Can you work these out from the drawing? Everything is in mm from the part's minimum corner. Give positions to 0.01 mm unless a question says otherwise; leave off trailing zeros. Order: outer loops, then holes, each group sorted by start corner. A loop starts at its lowest first (then second) coordinate and runs counter-clockwise, first axis right, second up. Notation, with made-up numbers: M -29.5,54.25 L -4.5,54.25 A25 ccw -4.5,80.25 Z; hole C 16.25,73.5 d4. An arc over 180 degrees is marked long. Answer as a JSON object with one key per item and string values.
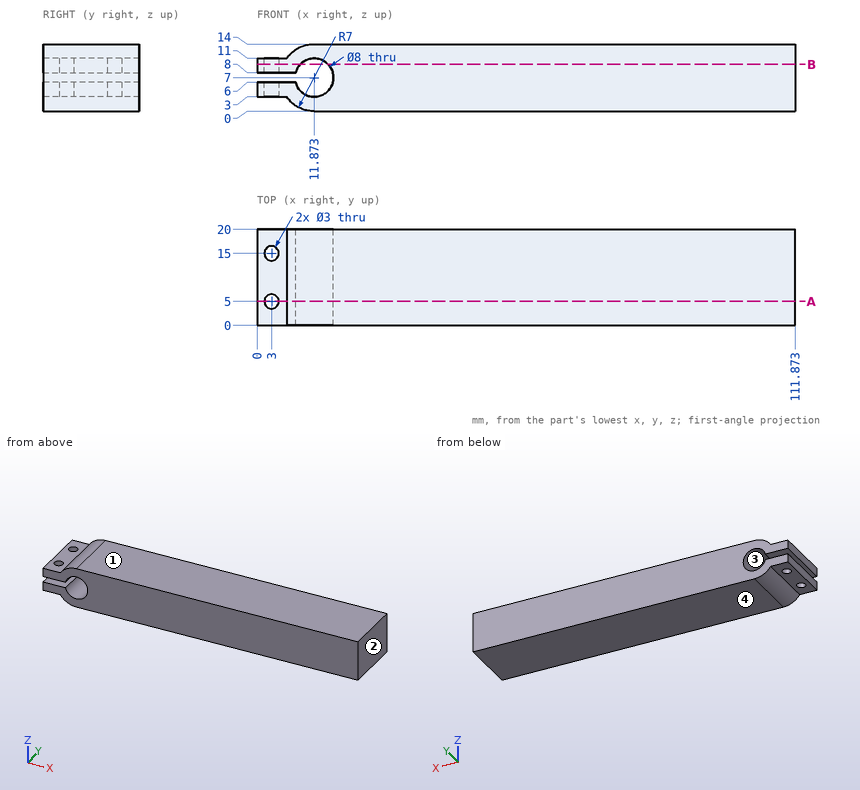
1) I need wall thicknesses on L1, parallel to Y at x = 3, z = 9.65; L2, parallel to Z at x = 14, y = 18.75; L3, parallel to X at y = 13.25, z = 7. Which ranges of each line are inside material? Lowest first, please.
Results found:
{"L1": "y = 0 to 3.5, 6.5 to 13.5, 16.5 to 20", "L2": "z = 0 to 3.61, 10.39 to 14", "L3": "x = 15.87 to 111.87"}
2) Thinking about a two-plate mould opening in Z: for the marked faces 1, 2, 3 and 4, which applies, pulls with the +Z half, pulls with the -Z half, needs draft (parallel to the pull), parting line crosses it, or undercut?
Results found:
{"face 1": "pulls with the +Z half", "face 2": "needs draft", "face 3": "undercut", "face 4": "pulls with the -Z half"}
3) I want a section at B-B on z = 9.75. Write out the boundary of the cut face in (x, y), and give its area (3 significant figures).
Results found:
{"outline": "M 0,0 L 8.97,0 L 8.97,20 L 0,20 Z; M 14.78,0 L 111.87,0 L 111.87,20 L 14.78,20 Z; hole C 3,5 d3; hole C 3,15 d3", "area": "2,110 mm²"}
4) I want a section at A-A on y = 5. Write out the boundary of the cut face in (x, z), and give its area (3 significant figures).
Results found:
{"outline": "M 0,3 L 1.5,3 L 1.5,6 L 0,6 Z; M 0,8 L 1.5,8 L 1.5,11 L 0,11 Z; M 4.5,3 L 6.13,3 A7 ccw 11.87,0 L 111.87,0 L 111.87,14 L 11.87,14 A7 ccw 6.13,11 L 4.5,11 L 4.5,8 L 8,8 A4 cw long 8,6 L 4.5,6 Z", "area": "1,440 mm²"}
5) I'm going to push flat-ended pins straight in: pin 1 Ø3.5 at (x, y) = (3, 5) entering from +Z; pin 2 Ø4 at (x, y) = (5.5, 5.5) entering from -Z; pin 3 Ø3 at (x, y) = (3, 6) entering from -Z. Where does each tip first touch, or does it pass through?
Results found:
{"pin 1": "stops at z = 11", "pin 2": "stops at z = 1.53", "pin 3": "stops at z = 3"}
